Part model, mm, in its own coordinate system. A direction names the side the tool comes from. Give positions to 0.01 mm unless a question says otherwise; leave off trailing zeros. Write each loop counter-clockwise with the first axis right and the second up, starting at its lowest first coordinate (ties: lowest second). Pieces come first, ordered by that corner, then holes. Notation, with made-up numbers: M -21,73.25 L 35,73.25 A19 cw 35,108.25 Z; hole C -15,-35.5 d1. An arc over 180 degrees is marked long. Answer as CSV lines item,"result". Start each with the question number.
1) Mould opens along X. For faces 1 (the flat face through (5.2, -2.5, 0)), 2 (the cylindrical face through (-11.99, 0.53, 2.46)), 3 (the cylindrical face through (0.07, -9.5, 2.46)) say: pulls with the +X half, pulls with the -X half, needs draft (parallel to the pull), parting line crosses it, or undercut.
2) Wall check: line 1 along X through (y, z) = (-0.5, 0.6); line 2 along X through (y, z) = (0.5, 4.2); line 3 along Y through (x, z) = (0.75, 4.7). Give the ranges that are in metal, low to high. Write a range as from..to.
3) Pin check, flat tips, straight feed: pin 1 Ø1.5 at (x, y) = (1.5, -3) entering from -Z; pin 2 Ø2.5 at (x, y) = (8, 0) entering from -Z; pin 3 Ø13.5 at (x, y) = (0, 0) entering from -Z; pin 4 Ø3 at (y, z) = (2, 3.5) entering from -X. Stop position of each tip, or through.
4) Tool access for faces 4 (the cylindrical face through (9.5, 0.07, 2.46)), 5 (the flat face through (-4, 2, 2.5)): list every direction of +Z, -Z, +X, -X, +Y, -Y with a clear straight run to the whole face (end or side of a thin tool).
5) Slice it at A-A, the plane y = 0. Give the cut face in (x, z), plus the area to 4 significant figures.
6) Slice it at C-C, the plane z = 3.4. Give the cut face in (x, y), plus the area to 3 significant figures.
7) Slice it at D-D, the plane x = 8.5. Give the cut face in (y, z).
```python
from build123d import *

# Parameters (mm, degrees)
F0_R            = 12
F1_DEPTH        = 5
F2_R            = 4
F3_DEPTH        = 5
F5_R            = 1.5
F6_DEPTH        = 5
F6_COPIES_COUNT = 4
F4_R            = 5.25
F7_DEPTH        = 2.5


# Not quite as in the source:
# - a pattern or mirror of a feature is missing from the dataset's text; its kind, count and spacing are read off the source's solid


with BuildPart() as f1:
    # F0 (on Top) → F1 (new body)
    with BuildSketch(Plane.XY):
        Circle(F0_R)
    extrude(amount=F1_DEPTH)

    # F2 (on face) → F3 (cut, through all)
    with BuildSketch(Plane(origin=(0, 0, 0), x_dir=(1, 0, 0), z_dir=(0, 0, -1))):
        Circle(F2_R)
    extrude(amount=-F3_DEPTH, mode=Mode.SUBTRACT)

    # F5 (on face) → F6 (cut, through all)
    with BuildSketch(Plane(origin=(0, 0, 0), x_dir=(1, 0, 0), z_dir=(0, 0, -1))):
        with Locations((-8, 0)):
            Circle(F5_R)
    f6 = extrude(amount=-F6_DEPTH, mode=Mode.SUBTRACT)

    # F6_copies: F6 ×4 about axis
    f6_copies_axis = Axis((0, 0, 0), (0, 0, 1))
    for i in range(1, F6_COPIES_COUNT):
        add(f6.rotate(f6_copies_axis, i * 360 / F6_COPIES_COUNT), mode=Mode.SUBTRACT)

    # F4 (on face) → F7 (cut)
    with BuildSketch(Plane(origin=(0, 0, 0), x_dir=(1, 0, 0), z_dir=(0, 0, -1))):
        Circle(F4_R)
    extrude(amount=-F7_DEPTH, mode=Mode.SUBTRACT)


solid = f1.part
```
Found:
1,face 1,"needs draft"
1,face 2,"parting line crosses it"
1,face 3,"undercut"
2,line 1,"-11.99..-9.41, -6.59..-5.23, 5.23..6.59, 9.41..11.99"
2,line 2,"-11.99..-9.41, -6.59..-3.97, 3.97..6.59, 9.41..11.99"
2,line 3,"-11.98..-9.3, -6.7..-3.93, 3.93..6.7, 9.3..11.98"
3,pin 1,"z = 2.5"
3,pin 2,"through"
3,pin 3,"z = 0"
3,pin 4,"x = -11.99"
4,face 4,"+Z, -Z"
4,face 5,"-Z"
5,outline,"M -12,0 L -9.5,0 L -9.5,5 L -12,5 Z; M -6.5,0 L -5.25,0 L -5.25,2.5 L -4,2.5 L -4,5 L -6.5,5 Z; M 4,2.5 L 5.25,2.5 L 5.25,0 L 6.5,0 L 6.5,5 L 4,5 Z; M 9.5,0 L 12,0 L 12,5 L 9.5,5 Z"
5,area,"43.75 mm²"
6,outline,"C 0,0 d24; hole C -8,0 d3; hole C 0,0 d8; hole C 0,-8 d3; hole C 0,8 d3; hole C 8,0 d3"
6,area,"374 mm²"
7,outline,"M -8.47,0 L -1.41,0 L -1.41,5 L -8.47,5 Z; M 1.41,0 L 8.47,0 L 8.47,5 L 1.41,5 Z"
